```python
from build123d import *

# Parameters (mm, degrees)
BOSS_EXTRUDE1_DEPTH = 12


with BuildPart() as part:
    # Sketch1 → Boss-Extrude1 (new body)
    with BuildSketch(Plane.XY):
        Polygon((-49.267596403, 5.5), (-50, 3.487737656), (-50, -5.5), (50, -5.5), (50, 3.25), (49.55556463, 3.25), (48.736631603, 5.5), (48.121775747, 5.5), (47.30284272, 3.25), (46.41397198, 3.25), (45.595038953, 5.5), (44.980183097, 5.5), (44.16125007, 3.25), (43.27237933, 3.25), (42.453446303, 5.5), (41.838590447, 5.5), (41.01965742, 3.25), (40.13078668, 3.25), (39.311853653, 5.5), (38.696997797, 5.5), (37.87806477, 3.25), (36.98919403, 3.25), (36.170261003, 5.5), (35.555405147, 5.5), (34.73647212, 3.25), (33.84760138, 3.25), (33.028668353, 5.5), (32.413812497, 5.5), (31.59487947, 3.25), (30.70600873, 3.25), (29.887075703, 5.5), (29.272219847, 5.5), (28.45328682, 3.25), (27.56441608, 3.25), (26.745483053, 5.5), (26.130627197, 5.5), (25.31169417, 3.25), (24.42282343, 3.25), (23.603890403, 5.5), (22.989034547, 5.5), (22.17010152, 3.25), (21.28123078, 3.25), (20.462297753, 5.5), (19.847441897, 5.5), (19.02850887, 3.25), (18.13963813, 3.25), (17.320705103, 5.5), (16.705849247, 5.5), (15.88691622, 3.25), (14.99804548, 3.25), (14.179112453, 5.5), (13.564256597, 5.5), (12.74532357, 3.25), (11.85645283, 3.25), (11.037519803, 5.5), (10.422663947, 5.5), (9.60373092, 3.25), (8.71486018, 3.25), (7.895927153, 5.5), (7.281071297, 5.5), (6.46213827, 3.25), (5.57326753, 3.25), (4.754334503, 5.5), (4.139478647, 5.5), (3.32054562, 3.25), (2.43167488, 3.25), (1.612741853, 5.5), (0.997885997, 5.5), (0.17895297, 3.25), (-0.70991777, 3.25), (-1.528850797, 5.5), (-2.143706653, 5.5), (-2.96263968, 3.25), (-3.85151042, 3.25), (-4.670443447, 5.5), (-5.285299303, 5.5), (-6.10423233, 3.25), (-6.99310307, 3.25), (-7.812036097, 5.5), (-8.426891953, 5.5), (-9.24582498, 3.25), (-10.13469572, 3.25), (-10.953628747, 5.5), (-11.568484603, 5.5), (-12.38741763, 3.25), (-13.27628837, 3.25), (-14.095221397, 5.5), (-14.710077253, 5.5), (-15.52901028, 3.25), (-16.41788102, 3.25), (-17.236814047, 5.5), (-17.851669903, 5.5), (-18.67060293, 3.25), (-19.55947367, 3.25), (-20.378406697, 5.5), (-20.993262553, 5.5), (-21.81219558, 3.25), (-22.70106632, 3.25), (-23.519999347, 5.5), (-24.134855203, 5.5), (-24.95378823, 3.25), (-25.84265897, 3.25), (-26.661591997, 5.5), (-27.276447853, 5.5), (-28.09538088, 3.25), (-28.98425162, 3.25), (-29.803184647, 5.5), (-30.418040503, 5.5), (-31.23697353, 3.25), (-32.12584427, 3.25), (-32.944777297, 5.5), (-33.559633153, 5.5), (-34.37856618, 3.25), (-35.26743692, 3.25), (-36.086369947, 5.5), (-36.701225803, 5.5), (-37.52015883, 3.25), (-38.40902957, 3.25), (-39.227962597, 5.5), (-39.842818453, 5.5), (-40.66175148, 3.25), (-41.55062222, 3.25), (-42.369555247, 5.5), (-42.984411103, 5.5), (-43.80334413, 3.25), (-44.69221487, 3.25), (-45.511147897, 5.5), (-46.126003753, 5.5), (-46.94493678, 3.25), (-47.83380752, 3.25), (-48.652740547, 5.5), align=None)
    extrude(amount=BOSS_EXTRUDE1_DEPTH)


solid = part.part
```
CAD build for the part. Positions are in the model's coordinates, mm. Coordinates: 2 decimals unless noted, no trailing zeros.
(1) Cut at A-A, the plane y = 4.5. Count the separate pieces of the cut face and the enclosed holes in it, and give its area (3 significant figures).
(2) Flat gauge pin, fed straight in: pin 1 (0.7 mm diameter, centred on x = 15.5, z = 6.5, fed in from +Y). Where does the tip first touch, or does it go through?
(3) Drill centre line: probe 1 along Y at (x, z) = (-32, 6.25). Where is it in solid material? Low to high.
(4) Two-plate mould, pull along X, no slides. Class faces 1 (the face through (-19.963, 4.359, 5.916)), 2 (the face through (50, -1, 6)): +X half, -X half, draft (parallel to the pull), parting line (faces both ways), or undercut.
Geometry says:
1. separate pieces: 32
1. enclosed holes: 0
1. area: 516 mm2
2. pin 1: stops at y = 3.25
3. probe 1: y = -5.5 to 3.25
4. face 1: undercut
4. face 2: +X half
